Autodesk Inventor part; units mm, degrees
ref_plane "YZ Plane" through (0, 0, 0) normal (1, 0, 0) x (0, 1, 0)
ref_plane "XZ Plane" through (0, 0, 0) normal (0, 1, 0) x (-1, 0, 0)
ref_plane "XY Plane" through (0, 0, 0) normal (0, 0, 1) x (1, 0, 0)
sketch "Sketch1" plane through (0, 0, 0) normal (0, 1, 0) x (-1, 0, 0)
  line L0 (0, 0) -> (6, 0)
  line L1 (6, 0) -> (6, -23)
  line L2 (6, -23) -> (0, -23)
  line L3 (0, -23) -> (0, 0)
  circle A0 centre (3, -1.85) radius 1
  circle A1 centre (3, -21.15) radius 1
  point P0 (3, 0)
  dimension "d0" = 6
  dimension "d1" = 23
  dimension "d2" = 2
  dimension "d3" = 2
  dimension "d4" = 19.3
  dimension "d5" = 1.85
  dimension "d6" = 3
extrude "Extrusion1" add sketch "Sketch1" along normal blind 1
sketch "Sketch2" plane through (0, 0, 0) normal (0, -1, 0) x (1, 0, 0)
  line L0 (-6, -23) -> (-6, 0)
  line L1 (0, 0) -> (0, -23)
  line L2 (-6, -4.5) -> (0, -4.5)
  line L3 (0, -4.5) -> (0, -18.5)
  line L4 (0, -18.5) -> (-6, -18.5)
  line L5 (-6, -18.5) -> (-6, -4.5)
  line L6 (-6, 0) -> (0, 0)
  point P0 (-3, -18.5)
  dimension "d9" = 14
  dimension "d10" = 4.5
extrude "Extrusion2" add sketch "Sketch2" along normal blind 5 contours L0 L2 L1 L4
sketch "Sketch3" plane through (0, 1, 0) normal (0, 1, 0) x (1, 0, 0)
  line L0 (-5, 6) -> (-1, 6)
  line L1 (-1, 6) -> (-1, 9.5)
  line L2 (-1, 9.5) -> (-5, 9.5)
  line L3 (-5, 9.5) -> (-5, 6)
  line L4 (-6, 23) -> (-6, 0)
  line L5 (-6, 0) -> (0, 0)
  dimension "d13" = 4
  dimension "d14" = 3.5
  dimension "d15" = 1
  dimension "d16" = 6
extrude "Extrusion3" add sketch "Sketch3" along normal blind 4
properties part number "SlideSwitchj"
Here's how the part is built. I have some questions about the finished solid (model axes, mm). A direction names the side the tool comes from. Coordinates: 2 decimals unless noted, no trailing zeros. Order: outer loops, then holes, each group sorted by start corner. A loop starts at its lowest first (then second) coordinate and runs counter-clockwise, first axis right, second up.
Item 1: I need wall thicknesses on probe 1 along Z at (x, y) = (-3, 0.6); probe 2 along Z at (x, y) = (-0.6, -1.25); probe 3 along Y at (x, z) = (-2.75, -12.25). Which ranges of each line are inside material? Lowest first, please.
Response values:
probe 1: z = -23 to -22.15, -20.15 to -2.85, -0.85 to 0
probe 2: z = -18.5 to -4.5
probe 3: y = -5 to 1
Item 2: Which directions (+Z, -Z, +X, -X, +Y, -Y) give clear straight access to the entire face, cutting with the end or side of a thin tool? Please do faces 4 (the face through (-3, 3, -9.5)), 5 (the face through (-2, 0, -20)), 6 (the face through (-5, 3, -8)).
Response values:
face 4: -Z, +X, -X, +Y
face 5: -Z, +X, -X, -Y
face 6: +Z, -Z, -X, +Y
Item 3: Thinking about a two-plate mould opening in Y: for faces 1 (the face through (-3, 5, -8)), 2 (the face through (-2.87, 0.49, -22.14)), 3 (the face through (-2, 0, -3)), which applies, pulls with the +Y half, pulls with the -Y half, needs draft (parallel to the pull), parting line crosses it, or undercut?
Response values:
face 1: pulls with the +Y half
face 2: needs draft
face 3: pulls with the -Y half
Item 4: If we section it at B-B, the plane x = -3: List the corners of the cut face in (y, z) for me.
Response values:
outline: (-5, -18.5) - (0, -18.5) - (0, -20.15) - (1, -20.15) - (1, -9.5) - (5, -9.5) - (5, -6) - (1, -6) - (1, -2.85) - (0, -2.85) - (0, -4.5) - (-5, -4.5) - close; (0, -23) - (1, -23) - (1, -22.15) - (0, -22.15) - close; (0, -0.85) - (1, -0.85) - (1, 0) - (0, 0) - close
Item 5: If we section it at C-C, the plane x = -4.35: List the corners of the cut face in (y, z) for me.
Response values:
outline: (-5, -18.5) - (0, -18.5) - (0, -23) - (1, -23) - (1, -9.5) - (5, -9.5) - (5, -6) - (1, -6) - (1, 0) - (0, 0) - (0, -4.5) - (-5, -4.5) - close
Item 6: If we section it at A-A, the plane z = -21.15: List the corners of the cut face in (x, y) for me.
Response values:
outline: (-6, 0) - (-4, 0) - (-4, 1) - (-6, 1) - close; (-2, 0) - (0, 0) - (0, 1) - (-2, 1) - close
Item 7: I'm going to push flat-ended pins straight in: pin 1 Ø2 at (x, y) = (-3, 3.5) entering from -Z; pin 2 Ø1.5 at (x, y) = (-3.5, -2.5) entering from -Z; pin 3 Ø1.8 at (x, z) = (-4.5, -14.5) entering from +Y. Where does each tip first touch, or does it pass through?
Response values:
pin 1: stops at z = -9.5
pin 2: stops at z = -18.5
pin 3: stops at y = 1
Item 8: If we section it at D-D, the plane z = -16.75: List the corners of the cut face in (x, y) for me.
Response values:
outline: (-6, -5) - (0, -5) - (0, 1) - (-6, 1) - close
